Can you work these out from the drawing? Everything is in mm from the part's minimum corner. A direction names the side the tool comes from. Coordinates: 2 decimals unless noted, no trailing zeros. Order: outer loops, then holes, each group sorted by start corner. A loop starts at its lowest first (then second) coordinate and runs counter-clockwise, first axis right, second up. Notation, with made-up numbers: M 83,59 L 124,59 A23 cw 124,87 Z; hole C 64.25,-21 d4. An arc over 180 degrees is marked long. Answer as a JSON object with one key per item and string values.
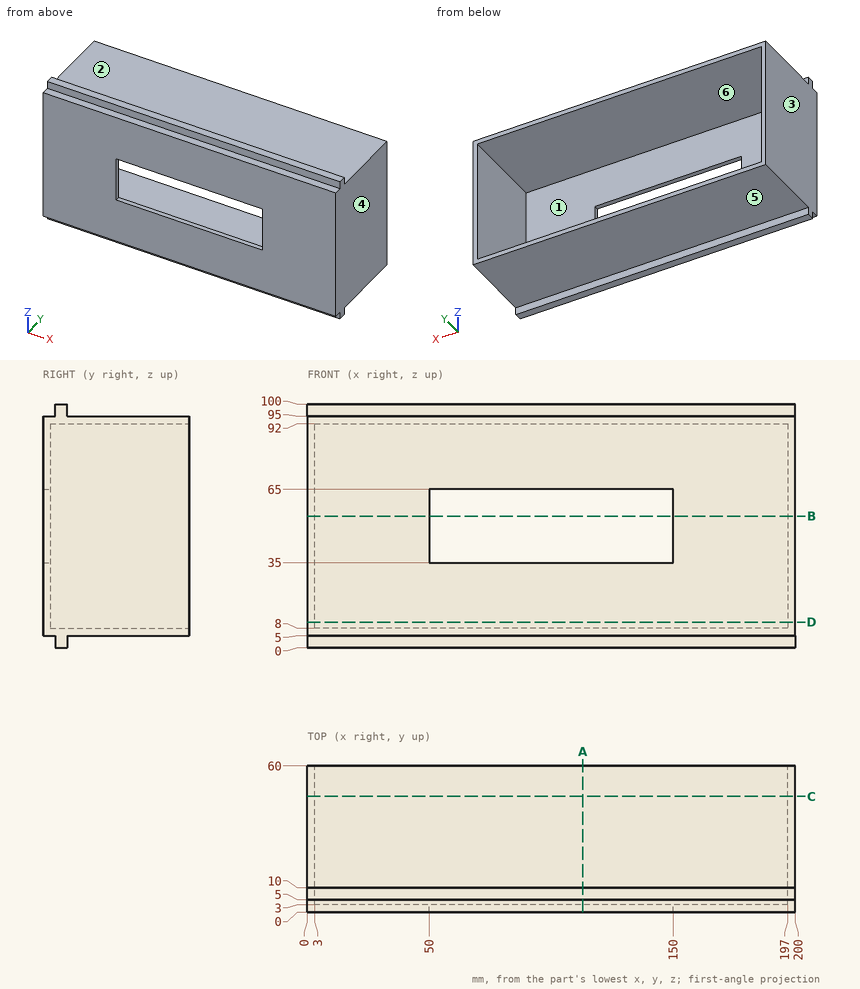
Item 1: Which directions (+Z, -Z, +X, -X, +Y, -Y) give clear straight access to the entire face, cutting with the end or side of a thin tool? Please do the marked faces 4, 5 and 6.
Answers follow:
{"face 4": "+Z, -Z, +X, +Y, -Y", "face 5": "-Z, +X, -X, +Y", "face 6": "+Y"}
Item 2: I want a section at C-C, the plane y = 47.5. Write out the boundary of the cut face in (x, z), plus the area to 3 significant figures.
Answers follow:
{"outline": "M 0,5 L 200,5 L 200,95 L 0,95 Z; hole M 3,8 L 197,8 L 197,92 L 3,92 Z", "area": "1,700 mm^2"}
Item 3: I'm going to push flat-ended pins straight in: pin 1 (8 mm diameter, centred on x = 114.5, y = 26.5, fed in from -Z); pin 2 (5.5 mm diameter, centred on x = 135, z = 2, fed in from -Y); pin 3 (1.5 mm diameter, centred on x = 105, z = 3, fed in from +Y). Where does each tip first touch, or does it pass through?
Answers follow:
{"pin 1": "stops at z = 5", "pin 2": "stops at y = 5", "pin 3": "stops at y = 10"}
Item 4: Please list where these lines run through material, in increasing order: line 1 (X direction, y = 33.5, z = 29); line 2 (Z direction, x = 165.5, y = 39.5); line 3 (Y direction, x = 37.5, z = 15).
Answers follow:
{"line 1": "x = 0 to 3, 197 to 200", "line 2": "z = 5 to 8, 92 to 95", "line 3": "y = 0 to 3"}
Item 5: I want a section at B-B, the plane z = 54. Write out the boundary of the cut face in (x, y).
Answers follow:
{"outline": "M 0,0 L 50,0 L 50,3 L 3,3 L 3,60 L 0,60 Z; M 150,0 L 200,0 L 200,60 L 197,60 L 197,3 L 150,3 Z"}
Item 6: I want a section at A-A, the plane x = 113. Write out the boundary of the cut face in (y, z).
Answers follow:
{"outline": "M 0,5 L 5,5 L 5,0 L 10,0 L 10,5 L 60,5 L 60,8 L 3,8 L 3,35 L 0,35 Z; M 0,65 L 3,65 L 3,92 L 60,92 L 60,95 L 10,95 L 10,100 L 5,100 L 5,95 L 0,95 Z"}
Item 7: If we mould it in two halves opening along X, with no side actions, what happens to the marked faces 1, 2 and 3? For each: pulls with the +X half, pulls with the -X half, needs draft (parallel to the pull), parting line crosses it, or undercut.
Answers follow:
{"face 1": "undercut", "face 2": "needs draft", "face 3": "pulls with the -X half"}
Item 8: I want a section at D-D, the plane z = 10.5. Write out the boundary of the cut face in (x, y).
Answers follow:
{"outline": "M 0,0 L 200,0 L 200,60 L 197,60 L 197,3 L 3,3 L 3,60 L 0,60 Z"}
